from build123d import *

# Parameters (mm, degrees)
F0_W          = 50
F0_H          = 50
F1_DEPTH      = 25
F1_DEPTH_BACK = 25
F2_R          = 12
F3_DEPTH      = 50
F4_R          = 12
F5_DEPTH      = 50
F6_R          = 12
F7_DEPTH      = 50


with BuildPart() as f1:
    # F0 (on Front) → F1 (new body, two sides)
    with BuildSketch(Plane.XZ) as f1_sk:
        Rectangle(F0_W, F0_H)
    extrude(amount=F1_DEPTH)
    extrude(f1_sk.sketch, amount=-F1_DEPTH_BACK)

    # F2 (on face) → F3 (cut)
    with BuildSketch(Plane.XZ.offset(25)):
        Circle(F2_R)
    extrude(amount=-F3_DEPTH, mode=Mode.SUBTRACT)

    # F4 (on face) → F5 (cut)
    with BuildSketch(Plane.XY.offset(25)):
        Circle(F4_R)
    extrude(amount=-F5_DEPTH, mode=Mode.SUBTRACT)

    # F6 (on face) → F7 (cut)
    with BuildSketch(Plane.YZ.offset(25)):
        Circle(F6_R)
    extrude(amount=-F7_DEPTH, mode=Mode.SUBTRACT)


solid = f1.part
Could you check a few things on this model? Use its own coordinates, in mm. Give positions to 0.01 mm unless a question says otherwise; leave off trailing zeros. Order: outer loops, then holes, each group sorted by start corner. A loop starts at its lowest first (then second) coordinate and runs counter-clockwise, first axis right, second up.
1. I need wall thicknesses on L1, parallel to X at y = 0, z = -15.75. Which ranges of the line are inside material? Lowest first, please.
Answers below:
L1: x = -25 to -12, 12 to 25
2. For pin 1 (19 mm diameter, centred on x = 0, y = 0, fed in from +Z), with a flat end and sliding along its axis, tell me the tip position at first contact or that it passes through.
Answers below:
pin 1: passes through
3. Suppose I cut it at A-A (x = 0). Write out the boundary of the cut face in (y, z), plus the area to 3 significant figures.
Answers below:
outline: (-25, -25) - (-12, -25) - (-12, -12) - (-25, -12) - close; (-25, 12) - (-12, 12) - (-12, 25) - (-25, 25) - close; (12, -25) - (25, -25) - (25, -12) - (12, -12) - close; (12, 12) - (25, 12) - (25, 25) - (12, 25) - close
area: 676 mm2
4. Suppose I cut it at C-C (y = -13). Write out the boundary of the cut face in (x, z), plus the area to 3 significant figures.
Answers below:
outline: (-25, -25) - (25, -25) - (25, 25) - (-25, 25) - close; hole circle Ø24 at (0, 0)
area: 2,050 mm2
5. Thinking about a two-plate mould opening in X: for faces 1 (the cylindrical face through (-8.844, 8.11, 18.693)), 2 (the flat face through (-11, 25, 6)), 3 (the flat face through (-25, -6, -11)), which applies, +X half, -X half, draft (parallel to the pull), parting line (faces both ways), or undercut?
Answers below:
face 1: undercut
face 2: draft
face 3: -X half
